Part print with two shaded views. Sizes in mm from the minimum x, y, z corner. A direction names the side the tool comes from. Coordinates: 2 decimals unless noted, no trailing zeros. Loops run counter-clockwise (first coordinate to the right, second up) from the corner with the lowest first, then second, coordinate; pieces in that order, holes last. Notation, with made-up numbers: (43.25, 38) -> (93.25, 38) arc R20 ccw to (93.25, 61) -> close; hole circle Ø6 at (86, 47.5). An arc over 180 degrees is marked (long way). Return JSON: item names as keys, results as strings. Group by question number.
(1) Flat gauge pins, fed straight in: pin 1 Ø2 at (y, z) = (7.5, 2) entering from -X; pin 2 Ø1 at (x, z) = (5, 1) entering from +Y; pin 3 Ø0.6 at (y, z) = (10.5, 2) entering from -X. Where does each tip first touch, or does it go through?
(2) Probe L1, parallel to Y at x = 5, z = 0.25; L2, parallel to X at y = 11.25, z = 3.1; L3, parallel to X at y = 8.5, z = 2.25. List the from-to ranges inside material, lowest first.
(3) Saw through at A-A on z = 1.75. Write the cut outline in (x, y).
(4) Tool access for the marked faces 1, 2 and 3: list every direction of +Z, -Z, +X, -X, +Y, -Y with a clear straight run to the whole face (end or side of a thin tool).
(5) Saw through at D-D on y = 4. Write the cut outline in (x, z), then the cut area to 3 significant figures.
(6) Saw through at B-B on y = 12.25. Write the cut outline in (x, z), then the cut area to 3 significant figures.
(7) Saw through at C-C on x = 5. Write the cut outline in (y, z).
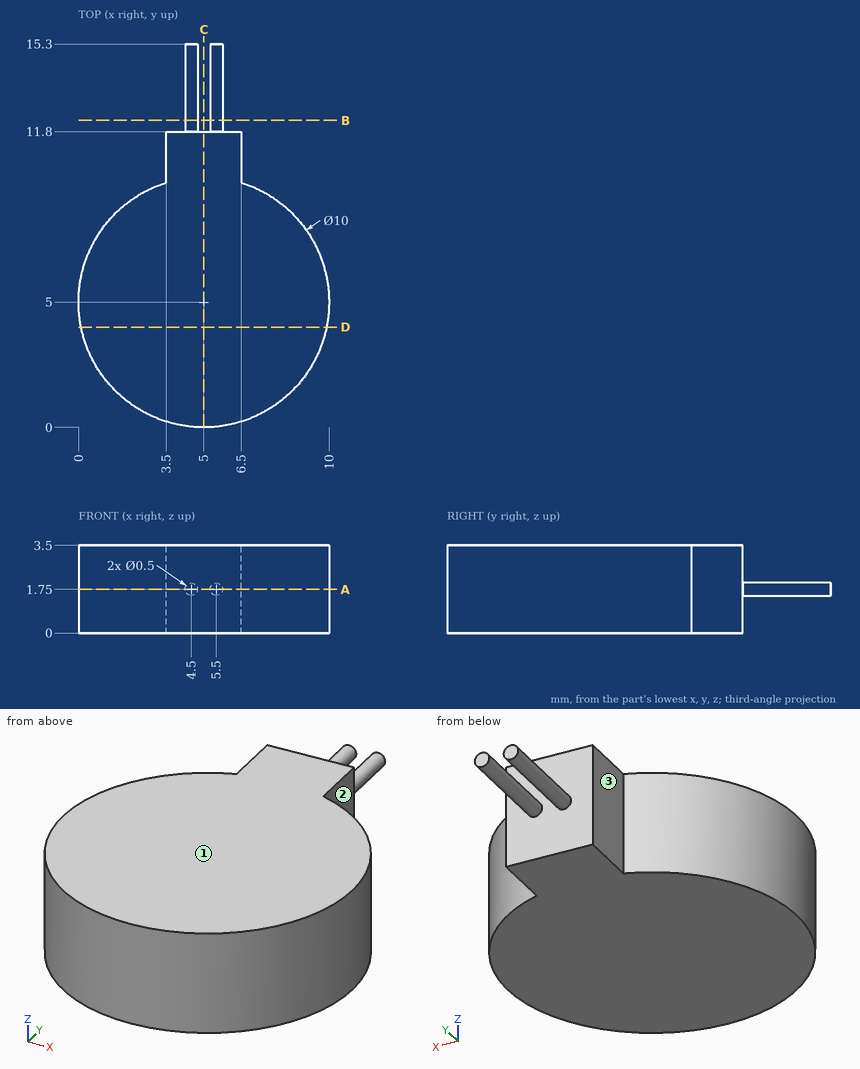
Geometry results:
{
 "1": {"pin 1": "x = 0.23", "pin 2": "y = 11.8", "pin 3": "x = 3.5"},
 "2": {"L1": "0 to 11.8", "L2": "3.5 to 6.5", "L3": "1.43 to 8.57"},
 "3": {"outline": "(3.5, 9.77) arc R5 ccw (long way) to (6.5, 9.77) -> (6.5, 11.8) -> (5.75, 11.8) -> (5.75, 15.3) -> (5.25, 15.3) -> (5.25, 11.8) -> (4.75, 11.8) -> (4.75, 15.3) -> (4.25, 15.3) -> (4.25, 11.8) -> (3.5, 11.8) -> close"},
 "4": {"face 1": "+Z, +X, -X, +Y, -Y", "face 2": "+Z, -Z, +X, +Y", "face 3": "+Z, -Z, -X, +Y"},
 "5": {"outline": "(0.1, 0) -> (9.9, 0) -> (9.9, 3.5) -> (0.1, 3.5) -> close", "area": "34.3 mm²"},
 "6": {"outline": "circle Ø0.5 at (4.5, 1.75); circle Ø0.5 at (5.5, 1.75)", "area": "0.393 mm²"},
 "7": {"outline": "(0, 0) -> (11.8, 0) -> (11.8, 3.5) -> (0, 3.5) -> close"}
}
